Design review of the part built by this model. Coordinates are the model's own, in mm. Coordinates: 2 decimals unless noted, no trailing zeros. Loops run counter-clockwise (first coordinate to the right, second up) from the corner with the lowest first, then second, coordinate; pieces in that order, holes last. Notation, with made-up numbers: (50, 54.5) -> (54, 54.5) arc R26 cw to (54, 79.5) -> close; hole circle Ø7 at (-14.5, 28.25). An arc over 180 degrees is marked (long way). One line per item, written item: value. Start each with the question number.
1. Add section C-C on y = 5.5. Write out the cut boundary in (x, z), plus the area to 3 significant figures.
2. Add section B-B on z = -3.5. Write out the cut boundary in (x, y).
3. Add section A-A on x = 0. Write out the cut boundary in (y, z), plus the area to 3 significant figures.
4. For probe 1 along Z at (x, y) = (0, 5); probe 2 along Z at (x, y) = (-2.5, 11); probe 3 along X at (y, z) = (7.75, 13), list the stretches that pass through material, from the lowest coordinate up.
5. Insertion check: pin 1 (6 mm diameter, centred on x = 2, y = 6.5, fed in from +Z). The pin has a flat end and moves straight along its axis. Give the tip position at first contact, or say it passes through.
6. Draft analysis for pull direction Z (two halves, no side actions). For faces 1 (the flat face through (0, 7, -25.4)), 2 (the cylindrical face through (2.581, 6.637, 11.623)), 3 (the flat face through (19.05, 7, -13)), 4 (the cylindrical face through (0.419, 6.637, 19.045)), state which applies: pulls with the +Z half, pulls with the -Z half, needs draft (parallel to the pull), parting line crosses it, or undercut.
7. Add section D-D on x = 13. Write out the cut boundary in (y, z), plus the area to 3 significant figures.
Autodesk Inventor part; units mm, degrees
ref_plane "YZ Plane" through (0, 0, 0) normal (1, 0, 0) x (0, 1, 0)
ref_plane "XZ Plane" through (0, 0, 0) normal (0, 1, 0) x (-1, 0, 0)
ref_plane "XY Plane" through (0, 0, 0) normal (0, 0, 1) x (1, 0, 0)
sketch "Sketch1" plane through (0, 0, 0) normal (0, 1, 0) x (-1, 0, 0)
  circle A0 centre (0, 0) radius 11.9062
  arc A1 (19.05, 0) -> (-19.05, 0) centre (0, 0) ccw
  line L0 (19.05, 0) -> (19.05, -25.4)
  line L1 (19.05, -25.4) -> (-19.05, -25.4)
  line L2 (-19.05, -25.4) -> (-19.05, 0)
  dimension "d0" = 23.8125
  dimension "d2" = 38.1
  dimension "d16" = 25.4
extrude "Extrusion1" add sketch "Sketch1" along normal blind 13.462
thread "Thread1"
properties part number "AcmeMountingFlange"
Worked answers:
1. outline: (-19.05, -25.4) -> (19.05, -25.4) -> (19.05, 0) arc R19.05 ccw to (-19.05, 0) -> close; hole circle Ø23.81 at (0, 0)
1. area: 1,090 mm²
2. outline: (-19.05, 0) -> (-11.38, 0) -> (-11.38, 13.46) -> (-19.05, 13.46) -> close; (11.38, 0) -> (19.05, 0) -> (19.05, 13.46) -> (11.38, 13.46) -> close
3. outline: (0, -25.4) -> (13.46, -25.4) -> (13.46, -11.91) -> (0, -11.91) -> close; (0, 11.91) -> (13.46, 11.91) -> (13.46, 19.05) -> (0, 19.05) -> close
3. area: 278 mm²
4. probe 1: z = -25.4 to -11.91, 11.91 to 19.05
4. probe 2: z = -25.4 to -11.64, 11.64 to 18.89
4. probe 3: x = -13.92 to 13.92
5. pin 1: stops at z = 19.05
6. face 1: pulls with the -Z half
6. face 2: undercut
6. face 3: needs draft
6. face 4: pulls with the +Z half
7. outline: (0, -25.4) -> (13.46, -25.4) -> (13.46, 13.92) -> (0, 13.92) -> close
7. area: 529 mm²
